Source: CAD feature listing. Evaluate the final solid. Frame: model axes, mm. Round coordinates to 2 decimals unless told otherwise and drop trailing zeros. Loops run counter-clockwise (first coordinate to the right, second up) from the corner with the lowest first, then second, coordinate; pieces in that order, holes last.
(1) First-contact query: pin 1 Ø4 at (x, y) = (171.45, 69.85) entering from -Z. Flat tip, straight axial feed; report the tip coordinate or a pass-through.
(2) Section C-C, the plane z = 2.45. Count the separate pieces of the cut face and the enclosed holes in it, plus the area to 3 significant figures.
(3) Section B-B, the plane x = 171.45. Return the cut outline in (y, z) (3 decimals).
(4) Section A-A, the plane y = 6.35. Return the cut outline in (x, z) (3 decimals), plus the area to 3 significant figures.
(5) Material intervals for probe 1 along Y at (x, z) = (6.35, 1.8); probe 2 along X at (y, z) = (50.5, 2.75); probe 3 along X at (y, z) = (50.8, 1.4), sorted ascending.
```python
from build123d import *

# Parameters (mm, degrees)
F0_W     = 177.8
F0_H     = 76.2
F3_DEPTH = 3.175
F4_DEPTH = 3.176
F5_D     = 4.3053
F6_D     = 9.5504


with BuildPart() as f3:
    # F0 (on Top) → F3 (new body)
    with BuildSketch(Plane.XY):
        with Locations((88.9, 38.1)):
            Rectangle(F0_W, F0_H)
    extrude(amount=F3_DEPTH)

    # F2 (on face) → F4 (cut, through all)
    with BuildSketch(Plane.XY):
        with BuildLine():
            ThreePointArc((47.0669316685, 16.2224972986), (50.0851940266, 16.6198590764), (49.6878322488, 19.6381214345))
            ThreePointArc((49.6878322488, 19.6381214345), (46.3399253491, 22.5741569859), (43.4038897977, 25.9220638856))
            ThreePointArc((43.4038897977, 25.9220638856), (40.3856274396, 26.3194256634), (39.9882656618, 23.3011633053))
            ThreePointArc((39.9882656618, 23.3011633053), (43.295618524, 19.5298501608), (47.0669316685, 16.2224972986))
        make_face()
        with BuildLine():
            ThreePointArc((88.3388878613, 16.2185305319), (91.3571502195, 16.6158923097), (90.9597884416, 19.6341546678))
            ThreePointArc((90.9597884416, 19.6341546678), (87.6113898152, 22.570621452), (84.674923031, 25.9190200784))
            ThreePointArc((84.674923031, 25.9190200784), (81.6566606729, 26.3163818563), (81.2592988951, 23.2981194981))
            ThreePointArc((81.2592988951, 23.2981194981), (84.5670829901, 19.5263146269), (88.3388878613, 16.2185305319))
        make_face()
        with BuildLine():
            ThreePointArc((129.6169316685, 16.2224972986), (132.6351940266, 16.6198590764), (132.2378322488, 19.6381214345))
            ThreePointArc((132.2378322488, 19.6381214345), (128.8899253491, 22.5741569859), (125.9538897977, 25.9220638856))
            ThreePointArc((125.9538897977, 25.9220638856), (122.9356274396, 26.3194256634), (122.5382656618, 23.3011633053))
            ThreePointArc((122.5382656618, 23.3011633053), (125.845618524, 19.5298501608), (129.6169316685, 16.2224972986))
        make_face()
    extrude(amount=F4_DEPTH, mode=Mode.SUBTRACT)

    # F5 (through all)
    with Locations(Plane(origin=(0, 0, 0), x_dir=(1, 0, 0), z_dir=(0, 0, -1))):
        with Locations((70.4115018816, -46.6457335184), (111.6865018816, -46.6457335184), (152.9615018816, -46.6457335184), (6.35, -69.85), (6.35, -6.35), (171.45, -69.85), (171.45, -6.35)):
            Hole(F5_D / 2)

    # F6 (through all)
    with Locations(Plane(origin=(0, 0, 0), x_dir=(1, 0, 0), z_dir=(0, 0, -1))):
        with Locations((47.625, -50.8), (88.9, -50.8), (130.175, -50.8)):
            Hole(F6_D / 2)


solid = f3.part
```
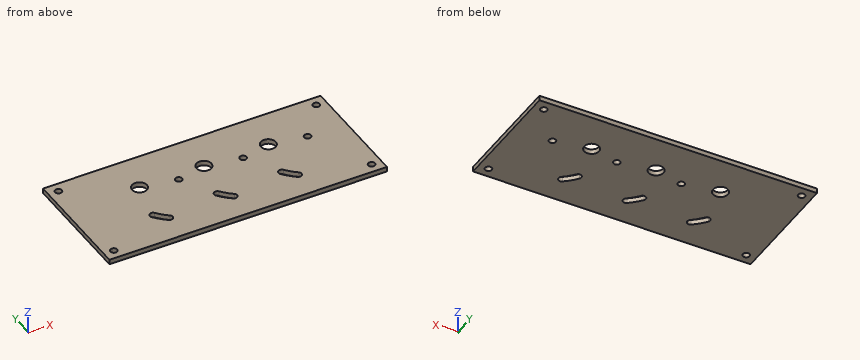
Output values:
1. pin 1: passes through
2. separate pieces: 1
2. enclosed holes: 13
2. area: 13,100 mm2
3. outline: (0, 0) - (4.197, 0) - (4.197, 3.175) - (0, 3.175) - close; (8.503, 0) - (67.697, 0) - (67.697, 3.175) - (8.503, 3.175) - close; (72.003, 0) - (76.2, 0) - (76.2, 3.175) - (72.003, 3.175) - close
4. outline: (0, 0) - (4.197, 0) - (4.197, 3.175) - (0, 3.175) - close; (8.503, 0) - (169.297, 0) - (169.297, 3.175) - (8.503, 3.175) - close; (173.603, 0) - (177.8, 0) - (177.8, 3.175) - (173.603, 3.175) - close
4. area: 537 mm2
5. probe 1: y = 0 to 4.2, 8.5 to 67.7, 72 to 76.2
5. probe 2: x = 0 to 42.86, 52.39 to 84.13, 93.67 to 125.41, 134.94 to 177.8
5. probe 3: x = 0 to 42.85, 52.4 to 84.12, 93.68 to 125.4, 134.95 to 177.8
